Work out the finished part from the listing and answer in its coordinate system (mm). Round coordinates to 2 decimals unless told otherwise and drop trailing zeros. Loops run counter-clockwise (first coordinate to the right, second up) from the corner with the lowest first, then second, coordinate; pieces in that order, holes last. Notation, with made-up numbers: (0, -34) - (35, -34) arc R23 ccw to (35, -9) - close; hole circle Ø1 at (35.25, -29). An arc over 180 degrees is marked (long way). Answer as CSV lines item,"result". Start each with the question number.
Q1. Section A-A on y = -1 is taken. Write down the section's boundary in (x, z) (3 decimals).
Q2. Straight lines are drawn through the part: L1, parallel to X at y = 1.2, z = 0 (3 decimals); L2, parallel to X at y = 3.75, z = 0; L3, parallel to Z at x = 0.15, y = -0.25. For each, find the intervals that lie inside material, in ascending order. Write a range as [from, to].
Q3. Section B-B on z = -1.4 is taken. Write down the section's boundary in (x, y), then the cut area to 3 significant figures.
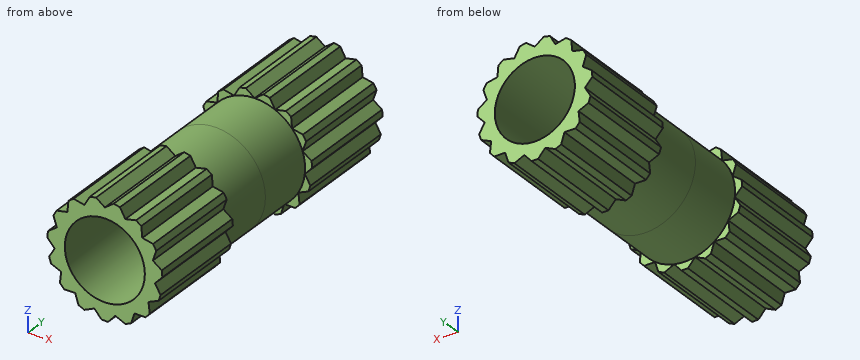
```python
from build123d import *

# Parameters (mm, degrees)
SKETCH1_R           = 1.575
SKETCH1_R_2         = 1.25
BOSS_EXTRUDE1_DEPTH = 5
BOSS_EXTRUDE2_DEPTH = 3.2


with BuildPart() as part:
    # Sketch1 → Boss-Extrude1 (new body)
    with BuildSketch(Plane(origin=(0, 0, 0), x_dir=(1, 0, 0), z_dir=(0, 1, 0))):
        Circle(SKETCH1_R)
        Circle(SKETCH1_R_2, mode=Mode.SUBTRACT)
    boss_extrude1 = extrude(amount=BOSS_EXTRUDE1_DEPTH)

    # Sketch2 → Boss-Extrude2 (add)
    with BuildSketch(Plane(origin=(0, 5, 0), x_dir=(1, 0, 0), z_dir=(0, 1, 0))):
        with BuildLine():
            ThreePointArc((-0.925761772, 1.274201766), (-0.640610213, 1.438834096), (-0.327460913, 1.540582471))
            Line((-0.327460913, 1.540582471), (-0.639640715, 1.682515901))
            Line((-0.639640715, 1.682515901), (-0.822349806, 1.601168572))
            Line((-0.822349806, 1.601168572), (-0.925761772, 1.274201766))
        make_face()
        with BuildLine():
            Line((-0.1, 1.797220076), (-0.327460913, 1.540582471))
            ThreePointArc((-0.327460913, 1.540582471), (0, 1.575), (0.327460913, 1.540582471))
            Line((0.327460913, 1.540582471), (0.1, 1.797220076))
            Line((0.1, 1.797220076), (-0.1, 1.797220076))
        make_face()
        with BuildLine():
            Line((0.639640715, 1.682515901), (0.327460913, 1.540582471))
            ThreePointArc((0.327460913, 1.540582471), (0.640610213, 1.438834096), (0.925761772, 1.274201766))
            Line((0.925761772, 1.274201766), (0.822349806, 1.601168572))
            Line((0.822349806, 1.601168572), (0.639640715, 1.682515901))
        make_face()
        with BuildLine():
            ThreePointArc((-1.363990011, 0.7875), (-1.1704531, 1.053880705), (-0.925761772, 1.274201766))
            Line((-0.925761772, 1.274201766), (-1.268681739, 1.276889441))
            Line((-1.268681739, 1.276889441), (-1.40250786, 1.128260476))
            Line((-1.40250786, 1.128260476), (-1.363990011, 0.7875))
        make_face()
        with BuildLine():
            Line((1.268681739, 1.276889441), (0.925761772, 1.274201766))
            ThreePointArc((0.925761772, 1.274201766), (1.1704531, 1.053880705), (1.363990011, 0.7875))
            Line((1.363990011, 0.7875), (1.40250786, 1.128260476))
            Line((1.40250786, 1.128260476), (1.268681739, 1.276889441))
        make_face()
        with BuildLine():
            ThreePointArc((-1.566371985, 0.16463233), (-1.497914013, 0.486701766), (-1.363990011, 0.7875))
            Line((-1.363990011, 0.7875), (-1.678356165, 0.650477198))
            Line((-1.678356165, 0.650477198), (-1.740159564, 0.460265894))
            Line((-1.740159564, 0.460265894), (-1.566371985, 0.16463233))
        make_face()
        with BuildLine():
            Line((1.678356165, 0.650477198), (1.363990011, 0.7875))
            ThreePointArc((1.363990011, 0.7875), (1.497914013, 0.486701766), (1.566371985, 0.16463233))
            Line((1.566371985, 0.16463233), (1.740159564, 0.460265894))
            Line((1.740159564, 0.460265894), (1.678356165, 0.650477198))
        make_face()
        with BuildLine():
            ThreePointArc((-1.497914013, -0.486701766), (-1.566371985, -0.16463233), (-1.566371985, 0.16463233))
            Line((-1.566371985, 0.16463233), (-1.797827562, -0.088408463))
            Line((-1.797827562, -0.088408463), (-1.77692187, -0.287312842))
            Line((-1.77692187, -0.287312842), (-1.497914013, -0.486701766))
        make_face()
        with BuildLine():
            Line((1.797827562, -0.088408463), (1.566371985, 0.16463233))
            ThreePointArc((1.566371985, 0.16463233), (1.566371985, -0.16463233), (1.497914013, -0.486701766))
            Line((1.497914013, -0.486701766), (1.77692187, -0.287312842))
            Line((1.77692187, -0.287312842), (1.797827562, -0.088408463))
        make_face()
        with BuildLine():
            ThreePointArc((-1.1704531, -1.053880705), (-1.363990011, -0.7875), (-1.497914013, -0.486701766))
            Line((-1.497914013, -0.486701766), (-1.606438242, -0.812007497))
            Line((-1.606438242, -0.812007497), (-1.506438242, -0.985212578))
            Line((-1.506438242, -0.985212578), (-1.1704531, -1.053880705))
        make_face()
        with BuildLine():
            ThreePointArc((-0.640610213, -1.438834096), (-0.925761772, -1.274201766), (-1.1704531, -1.053880705))
            Line((-1.1704531, -1.053880705), (-1.137281155, -1.395203059))
            Line((-1.137281155, -1.395203059), (-0.975477756, -1.512760109))
            Line((-0.975477756, -1.512760109), (-0.640610213, -1.438834096))
        make_face()
        with BuildLine():
            Line((1.606438242, -0.812007497), (1.497914013, -0.486701766))
            ThreePointArc((1.497914013, -0.486701766), (1.363990011, -0.7875), (1.1704531, -1.053880705))
            Line((1.1704531, -1.053880705), (1.506438242, -0.985212578))
            Line((1.506438242, -0.985212578), (1.606438242, -0.812007497))
        make_face()
        with BuildLine():
            ThreePointArc((0, -1.575), (-0.327460913, -1.540582471), (-0.640610213, -1.438834096))
            Line((-0.640610213, -1.438834096), (-0.471477825, -1.737155336))
            Line((-0.471477825, -1.737155336), (-0.275848305, -1.778737674))
            Line((-0.275848305, -1.778737674), (0, -1.575))
        make_face()
        with BuildLine():
            Line((1.137281155, -1.395203059), (1.1704531, -1.053880705))
            ThreePointArc((1.1704531, -1.053880705), (0.925761772, -1.274201766), (0.640610213, -1.438834096))
            Line((0.640610213, -1.438834096), (0.975477756, -1.512760109))
            Line((0.975477756, -1.512760109), (1.137281155, -1.395203059))
        make_face()
        with BuildLine():
            ThreePointArc((0.640610213, -1.438834096), (0.327460913, -1.540582471), (0, -1.575))
            Line((0, -1.575), (0.275848305, -1.778737674))
            Line((0.275848305, -1.778737674), (0.471477825, -1.737155336))
            Line((0.471477825, -1.737155336), (0.640610213, -1.438834096))
        make_face()
    boss_extrude2 = extrude(amount=-BOSS_EXTRUDE2_DEPTH)

    # Mirror1: Boss-Extrude1, Boss-Extrude2 across plane
    add(boss_extrude1.mirror(Plane.ZX))
    add(boss_extrude2.mirror(Plane.ZX))


solid = part.part
```
Findings:
1,outline,"circle Ø3.15 at (0, 0); hole circle Ø2.5 at (0, 0)"
2,L1,"x = [-1.575, -1.25], [1.25, 1.575]"
2,L2,"x = [-1.72, -1.25], [1.25, 1.72]"
2,L3,"z = [-1.57, -1.24], [1.24, 1.57]"
3,outline,"(-0.89, -5) - (0.89, -5) - (0.89, -1.8) - (0.72, -1.8) - (0.72, 1.8) - (0.89, 1.8) - (0.89, 5) - (-0.89, 5) - (-0.89, 1.8) - (-0.72, 1.8) - (-0.72, -1.8) - (-0.89, -1.8) - close"
3,area,"16.5 mm^2"
